For this review, take the finished solid that the model builds, in its own axes (mm). Face numbers are marked on the shaded views. Round coordinates to 2 decimals unless told otherwise and drop trailing zeros. Loops run counter-clockwise (first coordinate to the right, second up) from the corner with the lowest first, then second, coordinate; pieces in that order, holes last. Notation, with made-up numbers: (10.5, 59.25) -> (19.5, 59.25) arc R27 ccw to (19.5, 90.25) -> close; hole circle Ø4 at (74.5, 70.5). An arc over 180 degrees is marked (long way). Write each question's results on one line, items separated by ' | '.
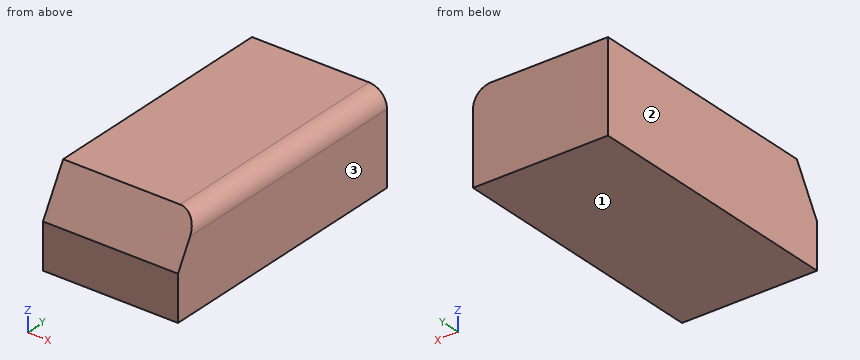
```python
from build123d import *

# Parameters (mm, degrees)
F0_W        = 38.1
F0_H        = 76.2
F1_DEPTH    = 25.4
F2_R        = 5.08
F3_T1_DEPTH = 98.731978168
F3_T6_ANGLE = 90


# Not quite as in the source:
# - a fillet or chamfer that OpenCascade refuses, or shapes differently, is made with other operations: its cross-section is extruded or revolved along the edge and cut away or added


with BuildPart() as f1:
    # F0 (on Top) → F1 (new body)
    with BuildSketch(Plane.XY):
        Rectangle(F0_W, F0_H)
    extrude(amount=F1_DEPTH)

    # F2
    f2_edges = [f1.edges().sort_by_distance(p)[0] for p in [
        (19.05, 0, 25.4),
    ]]
    fillet(f2_edges, radius=F2_R)

    # F3: chamfer of 12.7 x 7.3323484187 on 1 edges, made by hand

    # F3_s2 → F3_t1 (cut)
    with BuildSketch(Plane.YZ.offset(-51.905989084)):
        Polygon((-38.1, 12.7), (-30.7676515813, 25.4), (-38.1, 25.4), align=None)
    extrude(amount=F3_T1_DEPTH, mode=Mode.SUBTRACT)


with BuildPart() as f3_tool4:
    # F3_s5 → F3_t6 (revolve)
    with BuildSketch(Plane.XY.offset(20.32)):
        Polygon((13.97, -33.7005909488), (19.05, -30.7676515813), (19.05, -38.1), (13.97, -38.1), align=None)
    revolve(axis=Axis((13.97, -38.1, 20.32), (0, -1, 0)), revolution_arc=F3_T6_ANGLE)

    split(bisect_by=Plane(origin=(0, -34.074261314, 19.6727839421), x_dir=(1, 0, 0), z_dir=(0, -0.8660254038, 0.5)), keep=Keep.TOP)


with BuildPart() as f1_1:
    add(f1.part)

    # F3_t3: cut F3_tool4
    add(f3_tool4.part, mode=Mode.SUBTRACT)


solid = f1_1.part
```
1. Draft analysis for pull direction X (two halves, no side actions). For the marked faces 1, 2 and 3, state which applies: released by +X, released by -X, zero draft, split by the parting line, or undercut.
Values found:
face 1: zero draft | face 2: released by -X | face 3: released by +X
2. Consider section B-B (z = 17.75). State the section outline as (x, y) points.
Values found:
outline: (-19.05, -35.18) -> (19.05, -35.18) -> (19.05, 38.1) -> (-19.05, 38.1) -> close
3. Consider section A-A (x = -15.5). State the section outline as (y, z) points.
Values found:
outline: (-38.1, 0) -> (38.1, 0) -> (38.1, 25.4) -> (-30.77, 25.4) -> (-38.1, 12.7) -> close
4. To check wall thickness, follow probe 1 along Y at (x, z) = (9, 15); probe 2 along Y at (x, z) = (7, 13.25); probe 3 along Z at (x, y) = (9, -34). State the ranges of each line that lie inside material, in increasing order.
Values found:
probe 1: y = -36.77 to 38.1 | probe 2: y = -37.78 to 38.1 | probe 3: z = 0 to 19.8
